Source: CAD feature listing. Evaluate the final solid. Frame: model axes, mm. Coordinates: 2 decimals unless noted, no trailing zeros. Loops run counter-clockwise (first coordinate to the right, second up) from the corner with the lowest first, then second, coordinate; pieces in that order, holes last.
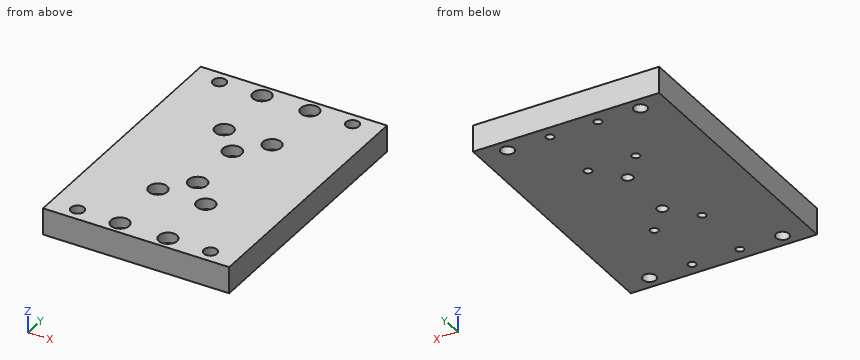
from build123d import *

# Parameters (mm, degrees)
SKETCH1_W           = 70
SKETCH1_H           = 100
BOSS_EXTRUDE1_DEPTH = 10
SKETCH2_R           = 2.5
CUT_EXTRUDE1_DEPTH  = 11
SKETCH3_R           = 1.5
CUT_EXTRUDE2_DEPTH  = 11
SKETCH4_R           = 3.45
CUT_EXTRUDE3_DEPTH  = 4
SKETCH5_R           = 2
CUT_EXTRUDE4_DEPTH  = 11
SKETCH6_R           = 3.5
CUT_EXTRUDE5_DEPTH  = 4


with BuildPart() as part:
    # Sketch1 → Boss-Extrude1 (new body)
    with BuildSketch(Plane.XY):
        Rectangle(SKETCH1_W, SKETCH1_H)
    extrude(amount=BOSS_EXTRUDE1_DEPTH)

    # Sketch2 → Cut-Extrude1 (cut, through all)
    with BuildSketch(Plane(origin=(0, 0, 0), x_dir=(-1, 0, 0), z_dir=(0, 0, -1))):
        with Locations((-25, 45)):
            Circle(SKETCH2_R)
        with Locations((25, 45)):
            Circle(SKETCH2_R)
        with Locations((-25, -45)):
            Circle(SKETCH2_R)
        with Locations((25, -45)):
            Circle(SKETCH2_R)
    extrude(amount=-CUT_EXTRUDE1_DEPTH, mode=Mode.SUBTRACT)

    # Sketch3 → Cut-Extrude2 (cut, through all)
    with BuildSketch(Plane(origin=(0, 0, 0), x_dir=(-1, 0, 0), z_dir=(0, 0, -1))):
        with Locations((9, 21)):
            Circle(SKETCH3_R)
        with Locations((9, 45)):
            Circle(SKETCH3_R)
        with Locations((-9, 21)):
            Circle(SKETCH3_R)
        with Locations((-9, 45)):
            Circle(SKETCH3_R)
        with Locations((9, -45)):
            Circle(SKETCH3_R)
        with Locations((9, -21)):
            Circle(SKETCH3_R)
        with Locations((-9, -45)):
            Circle(SKETCH3_R)
        with Locations((-9, -21)):
            Circle(SKETCH3_R)
    extrude(amount=-CUT_EXTRUDE2_DEPTH, mode=Mode.SUBTRACT)

    # Sketch4 → Cut-Extrude3 (cut)
    with BuildSketch(Plane.XY.offset(10)):
        with Locations((-9, 45)):
            Circle(SKETCH4_R)
        with Locations((-9, 21)):
            Circle(SKETCH4_R)
        with Locations((9, 21)):
            Circle(SKETCH4_R)
        with Locations((9, 45)):
            Circle(SKETCH4_R)
        with Locations((9, -21)):
            Circle(SKETCH4_R)
        with Locations((-9, -21)):
            Circle(SKETCH4_R)
        with Locations((-9, -45)):
            Circle(SKETCH4_R)
        with Locations((9, -45)):
            Circle(SKETCH4_R)
    extrude(amount=-CUT_EXTRUDE3_DEPTH, mode=Mode.SUBTRACT)

    # Sketch5 → Cut-Extrude4 (cut, through all)
    with BuildSketch(Plane.XY.offset(10)):
        with Locations((0, -11)):
            Circle(SKETCH5_R)
        with Locations((0, 11)):
            Circle(SKETCH5_R)
    extrude(amount=-CUT_EXTRUDE4_DEPTH, mode=Mode.SUBTRACT)

    # Sketch6 → Cut-Extrude5 (cut)
    with BuildSketch(Plane.XY.offset(10)):
        with Locations((0, 11)):
            Circle(SKETCH6_R)
        with Locations((0, -11)):
            Circle(SKETCH6_R)
    extrude(amount=-CUT_EXTRUDE5_DEPTH, mode=Mode.SUBTRACT)


solid = part.part
Q1. Section A-A, the plane y = -11. Return the cut outline in (x, z).
Q2. Section C-C, the plane z = 2.25. Count the separate pieces of the cut face and the enclosed holes in it, plus the area to 3 significant figures.
Q3. Section B-B, the plane x = -25. Return the cut outline in (y, z).
Q4. Section D-D, the plane y = 45. Return the cut outline in (x, z), plus the area to 3 significant figures.
Q5. Line query: line 1 along Y through (x, z) = (25, 7); line 2 along Y through (x, z) = (-9, 6.8); line 3 along Y through (x, z) = (0, 4.55). Output: solid intervals per line, ascending.
Q6. Contact query for flat-ended pins moving along their axis: pin 1 Ø5.5 at (x, y) = (-9, 20.5) entering from +Z; pin 2 Ø2.5 at (x, y) = (0, 11) entering from -Z. Output: stop coordinate, or through.
Derived:
1. outline: (-35, 0) - (-2, 0) - (-2, 6) - (-3.5, 6) - (-3.5, 10) - (-35, 10) - close; (2, 0) - (35, 0) - (35, 10) - (3.5, 10) - (3.5, 6) - (2, 6) - close
2. separate pieces: 1
2. enclosed holes: 14
2. area: 6,840 mm2
3. outline: (-50, 0) - (-47.5, 0) - (-47.5, 10) - (-50, 10) - close; (-42.5, 0) - (42.5, 0) - (42.5, 10) - (-42.5, 10) - close; (47.5, 0) - (50, 0) - (50, 10) - (47.5, 10) - close
4. outline: (-35, 0) - (-27.5, 0) - (-27.5, 10) - (-35, 10) - close; (-22.5, 0) - (-10.5, 0) - (-10.5, 6) - (-12.45, 6) - (-12.45, 10) - (-22.5, 10) - close; (-7.5, 0) - (7.5, 0) - (7.5, 6) - (5.55, 6) - (5.55, 10) - (-5.55, 10) - (-5.55, 6) - (-7.5, 6) - close; (10.5, 0) - (22.5, 0) - (22.5, 10) - (12.45, 10) - (12.45, 6) - (10.5, 6) - close; (27.5, 0) - (35, 0) - (35, 10) - (27.5, 10) - close
4. area: 509 mm2
5. line 1: y = -50 to -47.5, -42.5 to 42.5, 47.5 to 50
5. line 2: y = -50 to -48.45, -41.55 to -24.45, -17.55 to 17.55, 24.45 to 41.55, 48.45 to 50
5. line 3: y = -50 to -13, -9 to 9, 13 to 50
6. pin 1: stops at z = 6
6. pin 2: passes through
